```python
from build123d import *

# Parameters (mm, degrees)
SKETCH1_W           = 80
SKETCH1_H           = 80
BOSS_EXTRUDE1_DEPTH = 15
CUT_EXTRUDE2_DEPTH  = 8
CHAMFER3_SIZE       = 1.5
CUT_EXTRUDE3_DEPTH  = 115.127122105


with BuildPart() as part:
    # Sketch1 → Boss-Extrude1 (new body)
    with BuildSketch(Plane(origin=(0, 0, 0), x_dir=(1, 0, 0), z_dir=(0, 1, 0))):
        with Locations((40, 40)):
            Rectangle(SKETCH1_W, SKETCH1_H)
    extrude(amount=BOSS_EXTRUDE1_DEPTH)

    # Sketch3 → Cut-Extrude2 (cut)
    with BuildSketch(Plane(origin=(0, 15, 0), x_dir=(1, 0, 0), z_dir=(0, 1, 0))):
        Polygon((65, 80), (61.8, 80), (61.8, 18.2), (0, 18.2), (0, 15), (65, 15), align=None)
    extrude(amount=-CUT_EXTRUDE2_DEPTH, mode=Mode.SUBTRACT)

    # Chamfer3
    chamfer3_edges = [part.edges().sort_by_distance(p)[0] for p in [
        (65, 15, -47.5),
        (61.8, 15, -49.1),
        (30.9, 15, -18.2),
        (32.5, 15, -15),
    ]]
    chamfer(chamfer3_edges, length=CHAMFER3_SIZE)

    # Sketch4 → Cut-Extrude3 (cut, through all)
    with BuildSketch(Plane(origin=(0, 15, 0), x_dir=(1, 0, 0), z_dir=(0, 1, 0))):
        Polygon((0, 80), (50, 80), (0, 30), align=None)
    extrude(amount=-CUT_EXTRUDE3_DEPTH, mode=Mode.SUBTRACT)


solid = part.part
```
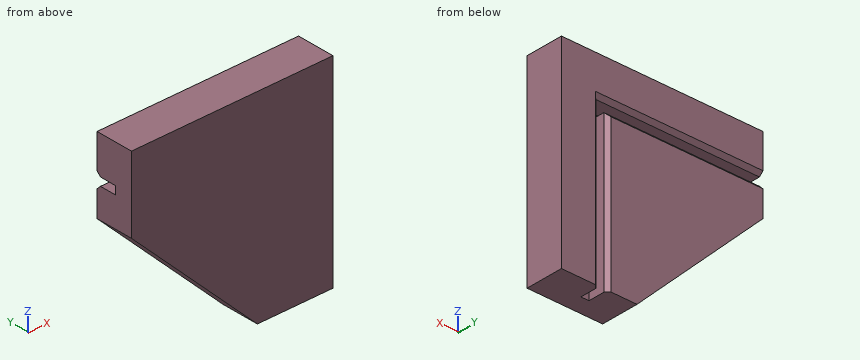
Model file for the job. Use its own axes, mm. Coordinates: 2 decimals unless noted, no trailing zeros. Loops run counter-clockwise (first coordinate to the right, second up) from the corner with the lowest first, then second, coordinate; pieces in that order, holes last. Notation, with made-up numbers: M -20.5,-37 L 15.5,-37 A22 cw 15.5,-4 Z; hole C 7.5,36 d8. An arc over 180 degrees is marked long. Use CSV: the item, a comma, the result in double quotes. Start each with the question number.
1. Band-saw the part on A-A, the plane y = 9.75. List the corners of the cut face in (x, z), then the cut area to 3 significant figures.
2. Flat gauge pins, fed straight in: pin 1 (1.5 mm diameter, centred on x = 72, y = 9.5, fed in from +Z); pin 2 (3 mm diameter, centred on x = 37, y = 11, fed in from -Z); pin 3 (3 mm diameter, centred on y = 11, z = -53.5, fed in from -X). Where does each tip first touch, or does it go through?
3. Probe probe 1 along Z at (x, y) = (59, 7.5); probe 2 along X at (y, z) = (13, -23); probe 3 along X at (y, z) = (11, -66.5). List the from-to ranges inside material, lowest first. Write a range as [from, to].
4. Band-saw the part on B-B, the plane z = -68.5. List the corners of the cut face in (x, y), then the cut area to 3 significant figures.
5. Band-saw the part on C-C, the plane x = 6.5. List the corners of the cut face in (y, z), then the cut area to 3 significant figures.
Entries:
1,outline,"M 0,-30 L 50,-80 L 61.8,-80 L 61.8,-18.2 L 0,-18.2 Z; M 0,-15 L 65,-15 L 65,-80 L 80,-80 L 80,0 L 0,0 Z"
1,area,"4,740 mm2"
2,pin 1,"stops at z = 0"
2,pin 2,"stops at z = -68.5"
2,pin 3,"stops at x = 22"
3,probe 1,"z = [-80, -18.2], [-15, 0]"
3,probe 2,"x = [0, 61.8], [65, 80]"
3,probe 3,"x = [36.5, 61.8], [65, 80]"
4,outline,"M 38.5,0 L 80,0 L 80,15 L 66.5,15 L 65,13.5 L 65,7 L 61.8,7 L 61.8,13.5 L 60.3,15 L 38.5,15 Z"
4,area,"595 mm2"
5,outline,"M 0,-36.5 L 15,-36.5 L 15,-19.7 L 13.5,-18.2 L 7,-18.2 L 7,-15 L 13.5,-15 L 15,-13.5 L 15,0 L 0,0 Z"
5,area,"520 mm2"
